Could you check a few things on this model? Use its own coordinates, in mm. Face numbers are marked on the shaded views. Round coordinates to 2 decimals unless told otherwise and drop trailing zeros. Loops run counter-clockwise (first coordinate to the right, second up) from the corner with the lowest first, then second, coordinate; pieces in that order, holes last. Notation, with made-up numbers: (43.25, 20) -> (88.25, 20) arc R21 cw to (88.25, 36) -> close; hole circle Ø3 at (4.25, 58). An arc over 180 degrees is marked (long way). Write each question's results on one line, items separated by ' | '.
from build123d import *

# Parameters (mm, degrees)
SKETCH_876_W           = 78
SKETCH_876_H           = 79
EXTRUDE_1660_DEPTH     = 18.2
SKETCH_1708_W          = 74.00014986
SKETCH_1708_H          = 75.0001524
SKETCH_1708_W_2        = 69.2
SKETCH_1708_H_2        = 50
SKETCH_1708_W_3        = 57.6
SKETCH_1708_H_3        = 43.2
LCD_DEPTH              = 2
LCD_2_OUTLINE_W        = 71.5
LCD_2_OUTLINE_H        = 52
LCD_2_OUTLINE_W_2      = 69.5
LCD_2_OUTLINE_H_2      = 50
LCD_2_DEPTH            = 2.6
LCD_3_DEPTH            = 2
SKETCH_9_R             = 1.55
SKETCH_9_R_2           = 1.00000254
PCB_DEPTH              = 4.6
USB_START              = 74.00015
SKETCH_11_W            = 1.6
SKETCH_11_H            = 5.5
SKETCH_11_W_2          = 3.4
SKETCH_11_H_2          = 10
SKETCH_11_W_3          = 2
SKETCH_11_H_3          = 15.11
SKETCH_11_H_4          = 6.51
USB_DEPTH              = 1.999925
CUT_EXTRUDE_7042_REACH = 91.005
SKETCH_12_W            = 12
SKETCH_12_H            = 2.4
FILLET_1_R             = 2


# Read off the part's stored shape, not the designer's step: LCD边框
with BuildPart() as part:
    # Sketch 876 → Extrude 1660 (new body)
    with BuildSketch(Plane.XY):
        with Locations((1.76392246, -1.007858704)):
            Rectangle(SKETCH_876_W, SKETCH_876_H)
        Polygon((-17.23611691, -38.507858704), (-14.23610929, -38.507858704), (38.76399739, -38.507858704), (38.76399739, -20.507823144), (38.76399739, 15.492250516), (38.76399739, 36.492293696), (-35.23615247, 36.492293696), (-35.23615247, -38.507858704), align=None, mode=Mode.SUBTRACT)
    extrude(amount=-EXTRUDE_1660_DEPTH)

    # Sketch 1708 → LCD (add)
    # profile 1 of 2: a face of its own
    with BuildSketch(Plane(origin=(0, 0, -18.2), x_dir=(-1, 0, 0), z_dir=(0, 0, -1))):
        with Locations((-1.76392246, -1.007782504)):
            Rectangle(SKETCH_1708_W, SKETCH_1708_H)
        with Locations((-1.76392246, -1.007858704)):
            Rectangle(SKETCH_1708_W_2, SKETCH_1708_H_2, mode=Mode.SUBTRACT)
    # profile 2 of 2: a face of its own
    with BuildSketch(Plane(origin=(0, 0, -18.2), x_dir=(-1, 0, 0), z_dir=(0, 0, -1))):
        with Locations((-1.76392246, -1.007858704)):
            Rectangle(SKETCH_1708_W_2, SKETCH_1708_H_2)
        with Locations((-4.96392246, -1.007858704)):
            Rectangle(SKETCH_1708_W_3, SKETCH_1708_H_3, mode=Mode.SUBTRACT)
    extrude(amount=-LCD_DEPTH)

    # LCD 2 outline → LCD 2 (add)
    with BuildSketch(Plane.XY.offset(-16.2)):
        with Locations((1.71392246, -1.007858704)):
            Rectangle(LCD_2_OUTLINE_W, LCD_2_OUTLINE_H)
        with Locations((1.71392246, -1.007858704)):
            Rectangle(LCD_2_OUTLINE_W_2, LCD_2_OUTLINE_H_2, mode=Mode.SUBTRACT)
    extrude(amount=LCD_2_DEPTH)

    # 草图7 → LCD 3 (add)
    with BuildSketch(Plane.XY.offset(-13.6)):
        Polygon((-23.904159925, -27.007858704), (-21.782839581, -24.886538361), (-22.489946362, -24.17943158), (-24.611266706, -26.300751923), align=None)
        Polygon((27.461068732, -27.007858704), (29.582389075, -24.886538361), (28.875282294, -24.17943158), (26.75396195, -26.300751923), align=None)
        Polygon((26.75396195, 24.285034514), (28.875282294, 22.163714171), (29.582389075, 22.870820952), (27.461068732, 24.992141296), align=None)
        Polygon((-24.611266706, 24.285034514), (-22.489946362, 22.163714171), (-21.782839581, 22.870820952), (-23.904159925, 24.992141296), align=None)
    extrude(amount=LCD_3_DEPTH)

    # 草图9 → PCB螺丝位 (add)
    # profile 1 of 4: a face of its own
    with BuildSketch(Plane.XY.offset(-16.2)):
        with Locations(Location((-30.179759278, 31.492141296, 0), (0, 0, 180))):
            Circle(SKETCH_9_R)
        with Locations(Location((-30.179759278, 31.492141296, 0), (0, 0, 180))):
            Circle(SKETCH_9_R_2, mode=Mode.SUBTRACT)
    # profile 2 of 4: a face of its own
    with BuildSketch(Plane.XY.offset(-16.2)):
        with Locations(Location((33.76398723, 31.492283536, 0), (0, 0, 180))):
            Circle(SKETCH_9_R)
        with Locations(Location((33.76398723, 31.492283536, 0), (0, 0, 180))):
            Circle(SKETCH_9_R_2, mode=Mode.SUBTRACT)
    # profile 3 of 4: a face of its own
    with BuildSketch(Plane.XY.offset(-16.2)):
        with Locations(Location((33.76398723, -33.507848544, 0), (0, 0, 180))):
            Circle(SKETCH_9_R)
        with Locations(Location((33.76398723, -33.507848544, 0), (0, 0, 180))):
            Circle(SKETCH_9_R_2, mode=Mode.SUBTRACT)
    # profile 4 of 4: a face of its own
    with BuildSketch(Plane.XY.offset(-16.2)):
        with Locations(Location((-30.23614231, -33.507848544, 0), (0, 0, 180))):
            Circle(SKETCH_9_R)
        with Locations(Location((-30.23614231, -33.507848544, 0), (0, 0, 180))):
            Circle(SKETCH_9_R_2, mode=Mode.SUBTRACT)
    extrude(amount=PCB_DEPTH)

    # 草图11 → 切除-USB边 (cut)
    with BuildSketch(Plane(origin=(-35.23615247, 0, 0), x_dir=(0, 0, -1), z_dir=(1, 0, 0)).offset(USB_START)):
        with Locations((9.2, -18.437706304)):
            Rectangle(SKETCH_11_W, SKETCH_11_H)
        with Locations((8.3, -7.007706304)):
            Rectangle(SKETCH_11_W_2, SKETCH_11_H_2)
        with Locations((9, 20.737293696)):
            Rectangle(SKETCH_11_W_3, SKETCH_11_H_3)
        with Locations((9.2, 4.207293696)):
            Rectangle(SKETCH_11_W, SKETCH_11_H_4)
    extrude(amount=USB_DEPTH, mode=Mode.SUBTRACT)

    # 草图12 → Cut-Extrude 7042 (cut, up to next)
    with BuildSketch(Plane.XZ.offset(-36.492293696), mode=Mode.PRIVATE) as cut_extrude_7042_sk1:
        with Locations((-18.89615247, -8.8)):
            Rectangle(SKETCH_12_W, SKETCH_12_H)
    cut_extrude_7042_tool1 = extrude(cut_extrude_7042_sk1.sketch, amount=-CUT_EXTRUDE_7042_REACH, mode=Mode.PRIVATE) & part.part
    add(cut_extrude_7042_tool1.solids().sort_by_distance((-18.896152, 36.492294, -8.8))[0], mode=Mode.SUBTRACT)

    # 圆角1
    fillet_1_edges = [part.edges().sort_by_distance(p)[0] for p in [
        (-37.23607754, -1.007858704, -18.2),
        (1.76392246, -40.507858704, -18.2),
        (40.76392246, -1.007858704, -18.2),
        (1.76392246, 38.492141296, -18.2),
    ]]
    fillet(fillet_1_edges, radius=FILLET_1_R)


solid = part.part
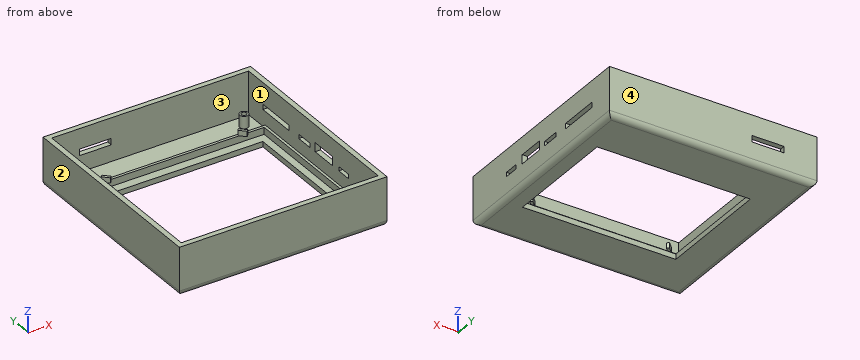
1) I need wall thicknesses on line 1 (X direction, y = -3.5, z = -15); line 2 (Y direction, x = 22, z = -16); line 3 (X direction, y = -12, z = -3.5). Which ranges of each line are inside material? Lowest first, please.
Model answer:
line 1: x = -37.24 to -35.24, -34.04 to -33.04, 36.46 to 37.46, 38.76 to 40.76 | line 2: y = -40.51 to -38.51, -27.01 to -26.01, 23.99 to 24.99, 36.49 to 38.49 | line 3: x = -37.24 to -35.24, 38.76 to 40.76
2) If we mould it in two halves opening along Y, with no side actions, what happens to the marked faces 1, 2, 3 and 4? For each: released by +Y, released by -Y, zero draft, split by the parting line, or undercut.
Model answer:
face 1: undercut | face 2: zero draft | face 3: undercut | face 4: released by +Y
3) I want a section at A-A, the plane x = -9. Write out the boundary of the cut face in (y, z).
Model answer:
outline: (-40.51, -16.2) arc R2 ccw to (-38.51, -18.2) -> (-22.61, -18.2) -> (-22.61, -16.2) -> (-26.01, -16.2) -> (-26.01, -13.6) -> (-27.01, -13.6) -> (-27.01, -16.2) -> (-38.51, -16.2) -> (-38.51, 0) -> (-40.51, 0) -> close; (20.59, -18.2) -> (36.49, -18.2) arc R2 ccw to (38.49, -16.2) -> (38.49, 0) -> (36.49, 0) -> (36.49, -16.2) -> (24.99, -16.2) -> (24.99, -13.6) -> (23.99, -13.6) -> (23.99, -16.2) -> (20.59, -16.2) -> close
4) I want a section at D-D, the plane z = -3.75. Write out the boundary of the cut face in (x, y).
Model answer:
outline: (-37.24, -40.51) -> (40.76, -40.51) -> (40.76, 38.49) -> (-37.24, 38.49) -> close; hole (-35.24, -38.51) -> (38.76, -38.51) -> (38.76, 36.49) -> (-35.24, 36.49) -> close
5) I'm going to push flat-ended pins straight in: pin 1 (3.5 mm diameter, centred on x = 33, y = 31, fed in from +Z); pin 2 (1.5 mm diameter, centred on x = -26, y = -22, fed in from +Z); pin 3 (0.5 mm diameter, centred on x = 10, y = 24.5, fed in from +Z). Where does each tip first touch, or does it pass through?
Model answer:
pin 1: stops at z = -11.6 | pin 2: stops at z = -16.2 | pin 3: stops at z = -13.6
6) I want a section at C-C, the plane z = -14.5. Give the number of separate pieces and of enclosed holes in the cut face, plus the area to 3 significant figures.
Model answer:
separate pieces: 6 | enclosed holes: 6 | area: 873 mm2
7) I want a section at B-B, the plane y = 2.5. Write out the boundary of the cut face in (x, z).
Model answer:
outline: (-37.24, -16.2) arc R2 ccw to (-35.24, -18.2) -> (-23.84, -18.2) -> (-23.84, -16.2) -> (-33.04, -16.2) -> (-33.04, -13.6) -> (-34.04, -13.6) -> (-34.04, -16.2) -> (-35.24, -16.2) -> (-35.24, 0) -> (-37.24, 0) -> close; (33.76, -18.2) -> (38.76, -18.2) arc R2 ccw to (40.76, -16.2) -> (40.76, -10) -> (38.76, -10) -> (38.76, -16.2) -> (37.46, -16.2) -> (37.46, -13.6) -> (36.46, -13.6) -> (36.46, -16.2) -> (33.76, -16.2) -> close; (38.76, -8.4) -> (40.76, -8.4) -> (40.76, 0) -> (38.76, 0) -> close
